```python
from build123d import *

# Parameters (mm, degrees)
BOSS_EXTRUDE1_DEPTH = 10
SKETCH2_R           = 50
CUT_EXTRUDE2_DEPTH  = 5
SKETCH3_W           = 307
SKETCH3_H           = 28
CUT_EXTRUDE3_DEPTH  = 5


with BuildPart() as part:
    # Sketch1 → Boss-Extrude1 (new body)
    with BuildSketch(Plane(origin=(0, 0, 0), x_dir=(1, 0, 0), z_dir=(0, 1, 0))):
        Polygon((175.101753381, 303.050121206), (-174.898226894, 303.167627278), (-349.999980275, 0.117506072), (-175.101753381, -303.050121206), (174.898226894, -303.167627278), (349.999980275, -0.117506072), align=None)
    extrude(amount=BOSS_EXTRUDE1_DEPTH)

    # Sketch2 → Cut-Extrude2 (cut)
    with BuildSketch(Plane(origin=(0, 10, 0), x_dir=(1, 0, 0), z_dir=(0, 1, 0))):
        with Locations(Location((-250.000009417, 0.041161845, 0), (0, 0, 270))):
            Circle(SKETCH2_R)
        with Locations(Location((-126.076603066, 215.895357646, 0), (0, 0, 270))):
            Circle(SKETCH2_R)
        with Locations(Location((249.999980275, 0, 0), (0, 0, 270))):
            Circle(SKETCH2_R)
        with Locations(Location((122.996764387, 217.697498973, 0), (0, 0, 270))):
            Circle(SKETCH2_R)
    extrude(amount=-CUT_EXTRUDE2_DEPTH, mode=Mode.SUBTRACT)

    # Sketch3 → Cut-Extrude3 (cut)
    with BuildSketch(Plane(origin=(0, 10, 0), x_dir=(1, 0, 0), z_dir=(0, 1, 0))):
        with Locations((0, 99.717508168)):
            Rectangle(SKETCH3_W, SKETCH3_H)
    extrude(amount=-CUT_EXTRUDE3_DEPTH, mode=Mode.SUBTRACT)


solid = part.part
```
Model file for the job. Use its own axes, mm. A direction names the side the tool comes from. Coordinates: 2 decimals unless noted, no trailing zeros. Loops run counter-clockwise (first coordinate to the right, second up) from the corner with the lowest first, then second, coordinate; pieces in that order, holes last. Notation, with made-up numbers: (-33, 38.25) - (-15, 38.25) arc R19 ccw to (-15, 48.25) - close; hole circle Ø10 at (86.5, 40.25). An arc over 180 degrees is marked (long way). Answer as a JSON object with one key per item and string values. Group by question number.
(1) Two-plate mould, pull along Z, no slides. Class faces 1 (the face through (-200.425, 7.535, -6.55)), 2 (the face through (-261.223, 4.93, -153.764)), 3 (the face through (-5, 10, -4)): released by +Z, released by -Z, zero draft, split by the parting line, or undercut.
(2) Cut at C-C (z = 174.5). Give the cut face in (x, y).
(3) Cut at A-A (y = 7.75). Give the cut face in (x, z).
(4) Tool access for faces 4 (the face through (261.223, 4.93, 153.764)), 5 (the face through (-125, 5, -217)): list every direction of +Z, -Z, +X, -X, +Y, -Y with a clear straight run to the whole face (end or side of a thin tool).
(5) Cut at B-B (x = -41). Give the cut face in (y, z), then the cut area to 3 significant figures.
(6) Flat gauge pins, fed straight in: pin 1 (2.5 mm diameter, centred on y = 7, z = -93.5, fed in from +X); pin 2 (4 mm diameter, centred on y = 6.5, z = 208, fed in from -X); pin 3 (1.5 mm diameter, centred on x = -152, y = 8.5, fed in from -Z). Where does each tip first touch, or does it go through?
(7) Probe line 1 along Z through (x, y) = (4.5, 8); line 2 along Z through (x, y) = (28, 4); line 3 along X through (y, z) = (8, -7). List the from-to ranges inside material, lowest first.
Geometry says:
{
 "1": {"face 1": "undercut", "face 2": "released by -Z", "face 3": "zero draft"},
 "2": {"outline": "(-249.26, 0) - (249.24, 0) - (249.24, 10) - (-249.26, 10) - close"},
 "3": {"outline": "(-350, -0.12) - (-174.9, -303.17) - (175.1, -303.05) - (350, 0.12) - (174.9, 303.17) - (-175.1, 303.05) - close; hole circle Ø100 at (-250, -0.04); hole circle Ø100 at (-126.08, -215.9); hole (-153.5, -113.72) - (153.5, -113.72) - (153.5, -85.72) - (-153.5, -85.72) - close; hole circle Ø100 at (123, -217.7); hole circle Ø100 at (250, 0)"},
 "4": {"face 4": "+Z, +X, +Y, -Y", "face 5": "+Y"},
 "5": {"outline": "(0, -303.12) - (10, -303.12) - (10, -113.72) - (5, -113.72) - (5, -85.72) - (10, -85.72) - (10, 303.1) - (0, 303.1) - close", "area": "5,920 mm^2"},
 "6": {"pin 1": "stops at x = 296.71", "pin 2": "stops at x = -231.09", "pin 3": "stops at z = -303.16"},
 "7": {"line 1": "z = -303.11 to -113.72, -85.72 to 303.11", "line 2": "z = -303.1 to 303.12", "line 3": "x = -346.02 to -299.51, -200.49 to 200.49, 299.51 to 345.89"}
}
